Check sheet for the modelled part. Datum: model origin and axes. Units: mm. Face numbers are marked on the shaded views. A direction names the side the tool comes from. Round coordinates to 2 decimals unless told otherwise and drop trailing zeros. Loops run counter-clockwise (first coordinate to the right, second up) from the corner with the lowest first, then second, coordinate; pieces in that order, holes last. Notation, with made-up numbers: (80, 0.25) - (93, 0.25) arc R15 cw to (93, 28.25) - close; hole circle Ø5 at (42, 6). An arc over 180 degrees is marked (long way). Put each result on its own line as item: value.
```python
from build123d import *

# Parameters (mm, degrees)
SKETCH_S_R                 = 9.525
BASE_FLANGE1_DEPTH         = 3.2639
F_1_4_0_2500_DOWEL_HOLE2_D = 6.35
EDGE_FLANGE1_DEPTH         = 63.5
F_1_2_CLEARANCE_HOLE1_D    = 13.89126
FILLET1_R                  = 12.7


# Sheet-metal steps are written as plain solids
with BuildPart() as part:
    # s → Base-Flange1 (new body)
    with BuildSketch(Plane.XY):
        with BuildLine():
            Line((31.75, -30.356048), (-31.75, -30.356048))
            Line((-31.75, -30.356048), (-141.763337817, -194.851484961))
            ThreePointArc((-141.763337817, -194.851484961), (-143.053340178, -220.94065371), (-120.65, -234.371929933))
            Line((-120.65, -234.371929933), (120.65, -234.371929933))
            ThreePointArc((120.65, -234.371929933), (143.053340178, -220.94065371), (141.763337817, -194.851484961))
            Line((141.763337817, -194.851484961), (31.75, -30.356048))
        make_face()
        with Locations((-120.65, -208.971929933)):
            Circle(SKETCH_S_R, mode=Mode.SUBTRACT)
        with Locations((120.65, -208.971929933)):
            Circle(SKETCH_S_R, mode=Mode.SUBTRACT)
    extrude(amount=-BASE_FLANGE1_DEPTH)

    # 1/4 (0.2500) Dowel Hole2 (through all)
    with Locations(Plane.XY):
        with Locations((-102.537139367, -167.610949699), (-89.341303231, -176.436227806), (-42.525248236, -77.879263975), (-29.3294121, -86.704542082), (29.3294121, -86.704542082), (42.525248236, -77.879263975), (89.341303231, -176.436227806), (102.537139367, -167.610949699)):
            Hole(F_1_4_0_2500_DOWEL_HOLE2_D / 2)

    # Edge-Flange1 section (across the edge) → Edge-Flange1 (add)
    with BuildSketch(Plane(origin=(31.75, -29.086048, 0), x_dir=(0, -1, 0), z_dir=(-1, 0, 0))):
        with BuildLine():
            Line((-3.2639, 1.27), (-3.2639, 47.5361))
            Line((-3.2639, 47.5361), (0, 47.5361))
            Line((0, 47.5361), (0, 1.27))
            ThreePointArc((0, 1.27), (0.371974388, 0.371974388), (1.27, 0))
            Line((1.27, 0), (1.27, -3.2639))
            ThreePointArc((1.27, -3.2639), (-1.935951435, -1.935951435), (-3.2639, 1.27))
        make_face()
    extrude(amount=EDGE_FLANGE1_DEPTH)

    # 1/2 Clearance Hole1 (through all)
    with Locations(Plane(origin=(0, -25.822148, 0), x_dir=(1, 0, 0), z_dir=(0, 1, 0))):
        with Locations((0, -22.1361)):
            Hole(F_1_2_CLEARANCE_HOLE1_D / 2)

    # Fillet1
    fillet1_edges = [part.edges().sort_by_distance(p)[0] for p in [
        (31.75, -27.454098, 47.5361),
        (-31.75, -27.454098, 47.5361),
    ]]
    fillet(fillet1_edges, radius=FILLET1_R)


solid = part.part
```
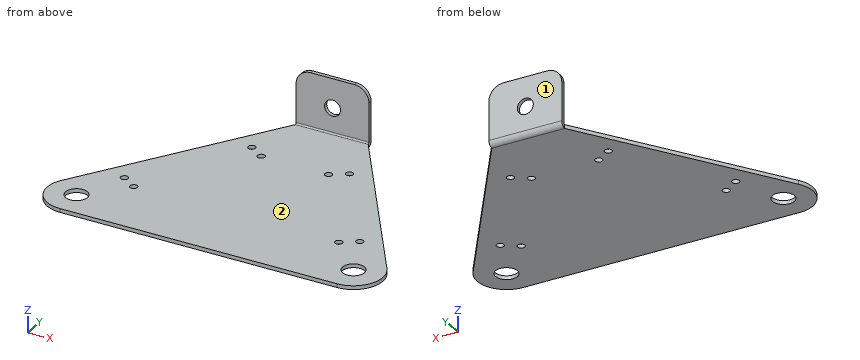
Item 1: Section check B-B on z = 9. Enter the section's corners in (x, y), then the cut area to 3 significant figures.
Filled sheet:
outline: (-31.75, -29.09) - (31.75, -29.09) - (31.75, -25.82) - (-31.75, -25.82) - close
area: 207 mm²
Item 2: Go/stop test with flat-tipped pins: pin 1 (8.5 mm diameter, centred on x = -42.53, y = -77.88, fed in from +Z); pin 2 (5 mm diameter, centred on y = -27.5, z = 20, fed in from -X); pin 3 (23 mm diameter, centred on x = 11.5, z = 14.5, fed in from -Y). Record where each tip stops, or that it passes through.
Filled sheet:
pin 1: z = 0
pin 2: x = -31.75
pin 3: y = -29.09
Item 3: Tool access check on the marked faces 1 and 2. Record the directions out of +Z, -Z, +X, -X, +Y, -Y that give a thin tool (end or side, any length) a straight path to the whole face; none if there is none.
Filled sheet:
face 1: +Z, -Z, +X, -X, +Y
face 2: +Z, +X, -X, -Y
Item 4: Section check A-A on x = 0. Enter the section's corners in (y, z).
Filled sheet:
outline: (-234.37, -3.26) - (-30.36, -3.26) arc R4.53 ccw to (-25.82, 1.27) - (-25.82, 15.19) - (-29.09, 15.19) - (-29.09, 1.27) arc R1.27 cw to (-30.36, 0) - (-234.37, 0) - close; (-29.09, 29.08) - (-25.82, 29.08) - (-25.82, 47.54) - (-29.09, 47.54) - close
Item 5: Thickness scan on line 1 (X direction, y = -204.5, z = -1); line 2 (Z direction, x = 51, y = -184); line 3 (Z direction, x = 0, y = -28.4). Record the ranges inside material, lowest first. Write a range as from..to.
Filled sheet:
line 1: -145.65..-129.06, -112.24..112.24, 129.06..145.65
line 2: -3.26..0
line 3: -2.82..15.19, 29.08..47.54
Item 6: Section check C-C on y = -103. Enter the section's corners in (x, z).
Filled sheet:
outline: (-80.33, -3.26) - (80.33, -3.26) - (80.33, 0) - (-80.33, 0) - close
